Could you check a few things on this drawing? It's one solid part, dimensions in mm from its lowest x, y, z. Round coordinates to 2 decimals unless told otherwise and drop trailing zeros. Write each loop counter-clockwise with the first axis right and the second up, starting at its lowest first coordinate (ties: lowest second). Pieces come first, ordered by that corner, then holes. Notation, with made-up numbers: (74.5, 66.5) -> (92.5, 66.5) arc R21 ccw to (92.5, 73.5) -> close; hole circle Ø6 at (21, -0.5). An arc over 180 degrees is marked (long way). Answer as CSV lines item,"result".
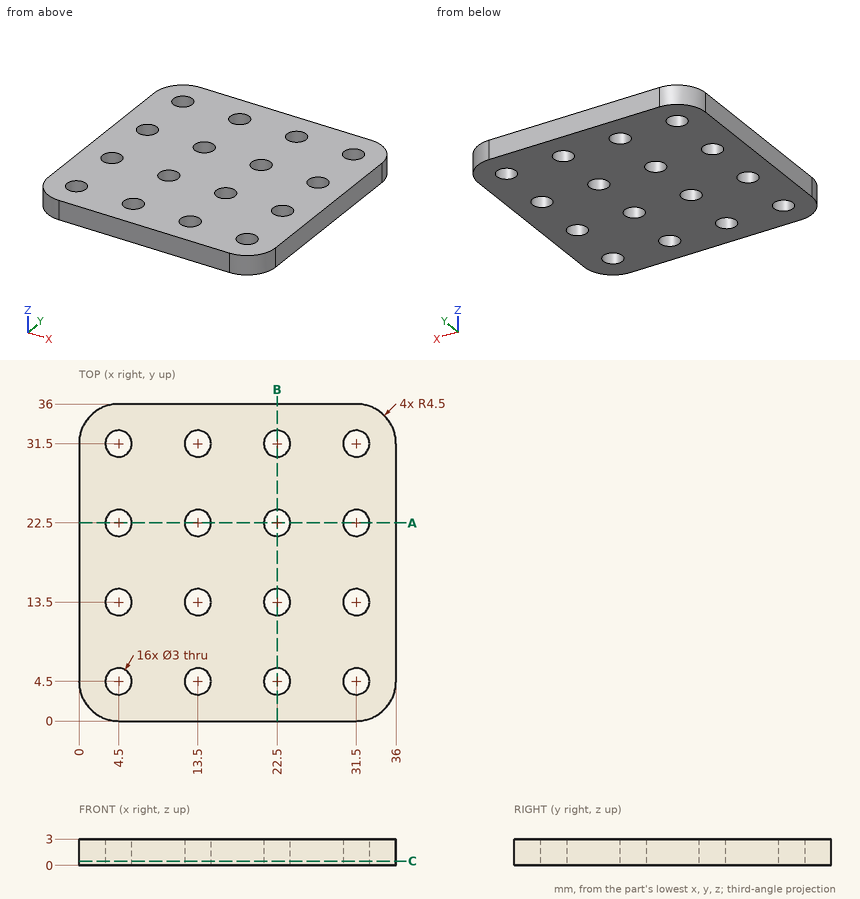
1. If I drill on line 1 (Y direction, x = 4.5, z = 0.95); line 2 (X direction, y = 12.5, z = 2.15), over which ranges is the centre line in solid material (lowest first)?
Numbers:
line 1,"y = 0 to 3, 6 to 12, 15 to 21, 24 to 30, 33 to 36"
line 2,"x = 0 to 3.38, 5.62 to 12.38, 14.62 to 21.38, 23.62 to 30.38, 32.62 to 36"
2. Suppose I cut it at A-A on y = 22.5. Please give me the cut outline in (x, z), and give its area (3 significant figures).
Numbers:
outline,"(0, 0) -> (3, 0) -> (3, 3) -> (0, 3) -> close; (6, 0) -> (12, 0) -> (12, 3) -> (6, 3) -> close; (15, 0) -> (21, 0) -> (21, 3) -> (15, 3) -> close; (24, 0) -> (30, 0) -> (30, 3) -> (24, 3) -> close; (33, 0) -> (36, 0) -> (36, 3) -> (33, 3) -> close"
area,"72.0 mm^2"
3. Suppose I cut it at C-C on z = 0.5. Count the separate pieces of the cut face and the enclosed holes in it, and give its area (3 significant figures).
Numbers:
separate pieces,"1"
enclosed holes,"16"
area,"1,170 mm^2"
4. For pin 1 Ø3.5 at (x, y) = (31.5, 4.5) entering from -Z, with a flat end and sliding along its axis, tell me the tip position at first contact or that it passes through.
Numbers:
pin 1,"stops at z = 0"
